```python
from build123d import *

# Parameters (mm, degrees)
EXTRUDE_1_DEPTH      = 3
SKETCH_2_R           = 5
EXTRUDE_2_DEPTH      = 40
SKETCH_3_R           = 7.5
EXTRUDE_3_DEPTH      = 3
CHAMFER_1_SIZE       = 3
EXTRUDE_4_DEPTH      = 40
EXTRUDE_5_DEPTH      = 30
EXTRUDE_5_DEPTH_BACK = 30
SKETCH_1_2_OUTSIDE_W = 83.046
SKETCH_1_2_OUTSIDE_H = 98.046
CUT_EXTRUDE_1_DEPTH  = 80.680612447
FILLET_1_R           = 2
FILLET_2_R           = 1
FILLET_3_R           = 2


with BuildPart() as part:
    # 草图1 → 凸台-拉伸1 (new body)
    with BuildSketch(Plane.XY):
        with BuildLine():
            Line((-14.576696831, 3.538348415), (-29.4, -57.528220211))
            ThreePointArc((-29.4, -57.528220211), (-29.028629911, -59.236212041), (-27.456440423, -60))
            Line((-27.456440423, -60), (27.456440423, -60))
            ThreePointArc((27.456440423, -60), (29.028629911, -59.236212041), (29.4, -57.528220211))
            Line((29.4, -57.528220211), (14.576696831, 3.538348415))
            ThreePointArc((14.576696831, 3.538348415), (0, 15), (-14.576696831, 3.538348415))
        make_face()
    extrude(amount=EXTRUDE_1_DEPTH)

    # 草图2 → 凸台-拉伸2 (add)
    with BuildSketch(Plane.XY.offset(3)):
        Circle(SKETCH_2_R)
    extrude(amount=EXTRUDE_2_DEPTH)

    # 草图3 → 凸台-拉伸3 (add)
    with BuildSketch(Plane.XY.offset(43)):
        Circle(SKETCH_3_R)
    extrude(amount=-EXTRUDE_3_DEPTH)

    # 倒角1
    # the kernel refuses this chamfer: 3 mm, written as the material it adds along each edge
    with BuildSketch(Plane(origin=(0, 0, 40), x_dir=(1, 0, 0), z_dir=(0, 1, 0))) as chamfer_1_piece_1_section:
        Polygon((5, CHAMFER_1_SIZE), (5 + CHAMFER_1_SIZE, 0), (5, 0), align=None)
    chamfer_1_piece_1 = revolve(axis=Axis((0, 0, 40), (0, 0, -1)), mode=Mode.PRIVATE)
    chamfer_1_piece_1 = chamfer_1_piece_1 & Plane(origin=(0, 0, 38.247274928), x_dir=(1, 0, 0), z_dir=(0, 0, 1)) * Cylinder(7.5, 32, mode=Mode.PRIVATE)
    add(chamfer_1_piece_1)
    with BuildSketch(Plane(origin=(0, 0, 3), x_dir=(1, 0, 0), z_dir=(0, -1, 0))) as chamfer_1_piece_2:
        Polygon((5 + CHAMFER_1_SIZE, 0), (5, CHAMFER_1_SIZE), (5, 0), align=None)
    revolve(axis=Axis((0, 0, 3), (0, 0, 1)))

    # 草图4 → 凸台-拉伸4 (add)
    with BuildSketch(Plane.XY.offset(3)):
        with BuildLine():
            Line((-29.271779789, -57), (29.271779789, -57))
            Line((29.271779789, -57), (29.4, -57.528220211))
            ThreePointArc((29.4, -57.528220211), (29.028629911, -59.236212041), (27.456440423, -60))
            Line((27.456440423, -60), (-27.456440423, -60))
            ThreePointArc((-27.456440423, -60), (-29.028629911, -59.236212041), (-29.4, -57.528220211))
            Line((-29.4, -57.528220211), (-29.271779789, -57))
        make_face()
    extrude(amount=EXTRUDE_4_DEPTH)

    # 草图6 → 凸台-拉伸5 (add, two sides: drawn at the far end of the back side and taken through both)
    with BuildSketch(Plane(origin=(0, 0, 0), x_dir=(0, 0, -1), z_dir=(1, 0, 0)).offset(-EXTRUDE_5_DEPTH_BACK)):
        Polygon((-43, -57), (-3, -55), (-3, -57), align=None)
    extrude(amount=EXTRUDE_5_DEPTH + EXTRUDE_5_DEPTH_BACK)

    # 草图1<2> outside → 切除-拉伸1 (cut, through all)
    with BuildSketch(Plane.XY):
        with Locations((0, -22.5)):
            Rectangle(SKETCH_1_2_OUTSIDE_W, SKETCH_1_2_OUTSIDE_H)
        with BuildLine():
            Line((-14.576696831, 3.538348415), (-29.4, -57.528220211))
            ThreePointArc((-29.4, -57.528220211), (-29.028629911, -59.236212041), (-27.456440423, -60))
            Line((-27.456440423, -60), (27.456440423, -60))
            ThreePointArc((27.456440423, -60), (29.028629911, -59.236212041), (29.4, -57.528220211))
            Line((29.4, -57.528220211), (14.576696831, 3.538348415))
            ThreePointArc((14.576696831, 3.538348415), (0, 15), (-14.576696831, 3.538348415))
        make_face(mode=Mode.SUBTRACT)
    extrude(amount=CUT_EXTRUDE_1_DEPTH, mode=Mode.SUBTRACT)

    # 圆角1
    fillet_1_edges = [part.edges().sort_by_distance(p)[0] for p in [
        (0, -55, 3),
    ]]
    fillet(fillet_1_edges, radius=FILLET_1_R)

    # 圆角2
    # the kernel refuses this fillet: 1 mm, written as the material it takes off along each edge
    with BuildSketch(Plane(origin=(27.456440423, -58, 43), x_dir=(0.971779788708135, 0.23588989435406618, 0), z_dir=(-0.23588989435406618, 0.971779788708135, 0))) as fillet_2_piece_1:
        with BuildLine():
            CenterArc((2 - FILLET_2_R, FILLET_2_R), FILLET_2_R, 270, 90)
            Line((2, FILLET_2_R), (2, 0))
            Line((2, 0), (2 - FILLET_2_R, 0))
        make_face()
    revolve(axis=Axis((27.456440423, -58, 43), (0, 0, -1)), revolution_arc=103.644084795, mode=Mode.SUBTRACT)
    with BuildSketch(Plane(origin=(27.456440423, -60, 43), x_dir=(0, 1, 0), z_dir=(-1, 0, 0))) as fillet_2_piece_2:
        with BuildLine():
            CenterArc((FILLET_2_R, FILLET_2_R), FILLET_2_R, 180, 90)
            Line((0, FILLET_2_R), (0, 0))
            Line((0, 0), (FILLET_2_R, 0))
        make_face()
    extrude(amount=54.912880845, mode=Mode.SUBTRACT)
    with BuildSketch(Plane(origin=(-27.456440423, -58, 43), x_dir=(0, -1, 0), z_dir=(1, 0, 0))) as fillet_2_piece_3:
        with BuildLine():
            CenterArc((2 - FILLET_2_R, FILLET_2_R), FILLET_2_R, 270, 90)
            Line((2, FILLET_2_R), (2, 0))
            Line((2, 0), (2 - FILLET_2_R, 0))
        make_face()
    revolve(axis=Axis((-27.456440423, -58, 43), (0, 0, -1)), revolution_arc=103.644084795, mode=Mode.SUBTRACT)
    with BuildSketch(Plane(origin=(-31.649902838, -57, 43), x_dir=(0, 0.049937616943894474, -0.9987523388778445), z_dir=(1, 0, 0))) as fillet_2_piece_4:
        with BuildLine():
            CenterArc((FILLET_2_R * 0.951249219725, -FILLET_2_R), FILLET_2_R, 90, 87.137594774)
            Line((-FILLET_2_R * 0.0475031191528, -FILLET_2_R * 0.950062383056), (0, 0))
            Line((0, 0), (FILLET_2_R * 0.951249219725, 0))
        make_face()
    extrude(amount=63.299805676, mode=Mode.SUBTRACT)
    with BuildSketch(Plane(origin=(-29.4, -57.528220211, 43), x_dir=(0, 0, -1), z_dir=(0.23588989435405947, 0.9717797887081366, 0)), Plane(origin=(28.682055053, -54.570550528, 43), x_dir=(0, 0, -1), z_dir=(0.2358898943540625, -0.971779788708136, 0))) as fillet_2_piece_5:
        with BuildLine():
            CenterArc((FILLET_2_R, -FILLET_2_R), FILLET_2_R, 90, 90)
            Line((0, -FILLET_2_R), (0, 0))
            Line((0, 0), (FILLET_2_R, 0))
        make_face()
    extrude(amount=3.043559577, mode=Mode.SUBTRACT)

    # 圆角3
    fillet_3_edges = [part.edges().sort_by_distance(p)[0] for p in [
        (-7.5, 0, 43),
    ]]
    fillet(fillet_3_edges, radius=FILLET_3_R)


solid = part.part
```
The listing builds one solid part. Answer for the finished solid, in the listing's coordinates (mm). A direction names the side the tool comes from. Coordinates: 2 decimals unless noted, no trailing zeros. Loops run counter-clockwise (first coordinate to the right, second up) from the corner with the lowest first, then second, coordinate; pieces in that order, holes last. Notation, with made-up numbers: (-31.75, -2.75) -> (12.25, -2.75) arc R23 ccw to (12.25, 29.25) -> close; hole circle Ø11 at (40.25, -26.75). An arc over 180 degrees is marked (long way). Return JSON: item names as keys, results as strings. Group by question number.
(1) Determine the mould class of faces 4 (the conical face through (-1.115, -5.023, 5.854)), 5 (the flat face through (0, -30, 0)), 6 (the cylindrical face through (29.04, -59.22, 20.71)) for opening direction Y: released by +Y, released by -Y, zero draft, split by the parting line, or undercut.
(2) Given pin 1 Ø17 at (x, y) = (10.5, -30.5) entering from +Z; pin 2 Ø5 at (x, z) = (-21.5, 32) entering from +Y (3 decimals); pin 3 Ø6 at (y, z) = (-6, 26.5) entering from +X, each flat-ended and moving along its own axis, determine where each tip first touches the part or whether it passes through.
(3) A cutting plane is placed at C-C on y = 0. Write down the section's boundary in (x, z).
(4) A cutting plane is placed at A-A on z = 33.5. Write down the section's boundary in (x, y) (3 decimals).
(5) Find the intervals of material crossed by probe 1 along Z at (x, y) = (-8.5, -38); probe 2 along Z at (x, y) = (-6, -3); probe 3 along Y at (x, z) = (-4, 19), in increasing order. Write a range as from..to.
(6) Which of the six approach directions +Z, -Z, +X, -X, +Y, -Y give full straight-line access (tool end or side, diameter ignored) to faces 1 (the cylindrical face through (0.403, -54.491, 3.566)), 2 (the conical face through (4.8, 2, 37.2)), 3 (the cylindrical face through (-7.493, 0.33, 40.26))?
(7) A cutting plane is placed at D-D on x = -9. Write down the section's boundary in (y, z) (1 decimal), and give its area (3 significant figures).
(8) A cutting plane is placed at B-B on x = 0. Write down the section's boundary in (y, z) (1 decimal), and give its area (3 significant figures).
The answers:
{
 "1": {"face 4": "undercut", "face 5": "zero draft", "face 6": "split by the parting line"},
 "2": {"pin 1": "stops at z = 3", "pin 2": "stops at y = -56.325", "pin 3": "stops at x = 4"},
 "3": {"outline": "(-15.44, 0) -> (15.44, 0) -> (15.44, 3) -> (8, 3) -> (5, 6) -> (5, 37) -> (7.5, 39.5) -> (7.5, 41) arc R2 ccw to (5.5, 43) -> (-5.5, 43) arc R2 ccw to (-7.5, 41) -> (-7.5, 39.5) -> (-5, 37) -> (-5, 6) -> (-8, 3) -> (-15.44, 3) -> close"},
 "4": {"outline": "(-29.4, -57.528) arc R2 ccw to (-27.456, -60) -> (27.456, -60) arc R2 ccw to (29.4, -57.528) -> (29.156, -56.525) -> (-29.156, -56.525) -> close; circle Ø10 at (0, 0)"},
 "5": {"probe 1": "z = 0..3", "probe 2": "z = 0..4.29, 38.71..42.59", "probe 3": "y = -60..-55.8, -3..3"},
 "6": {"face 1": "+Z, +X, -X", "face 2": "none", "face 3": "+Z"},
 "7": {"outline": "(-60, 0) -> (12, 0) -> (12, 3) -> (-53.1, 3) arc R2 cw to (-55.1, 4.9) -> (-57, 42) arc R1 ccw to (-58, 43) -> (-59, 43) arc R1 ccw to (-60, 42) -> close", "area": "376 mm^2"},
 "8": {"outline": "(-60, 0) -> (15, 0) -> (15, 3) -> (8, 3) -> (5, 6) -> (5, 37) -> (7.5, 39.5) -> (7.5, 41) arc R2 ccw to (5.5, 43) -> (-5.5, 43) arc R2 ccw to (-7.5, 41) -> (-7.5, 39.5) -> (-5, 37) -> (-5, 6) -> (-8, 3) -> (-53.1, 3) arc R2 cw to (-55.1, 4.9) -> (-57, 42) arc R1 ccw to (-58, 43) -> (-59, 43) arc R1 ccw to (-60, 42) -> close", "area": "816 mm^2"}
}
